For this review, take the finished solid that the model builds, in its own axes (mm). Round coordinates to 2 decimals unless told otherwise and drop trailing zeros. Order: outer loops, then holes, each group sorted by start corner. A loop starts at its lowest first (then second) coordinate and runs counter-clockwise, first axis right, second up. Notation, with made-up numbers: M 2.5,-23 L 6.5,-23 A12 ccw 6.5,-7 Z; hole C 81.25,-35 d2. An arc over 180 degrees is marked long. Write item = value, one per line. Start each with the question number.
from build123d import *

# Parameters (mm, degrees)
SKETCH1_R           = 109
BOSS_EXTRUDE1_DEPTH = 5
SKETCH2_R           = 114
SKETCH2_R_2         = 109
BOSS_EXTRUDE2_DEPTH = 105.1
SKETCH3_R           = 114
BOSS_EXTRUDE3_DEPTH = 5


with BuildPart() as part:
    # Sketch1 → Boss-Extrude1 (new body)
    with BuildSketch(Plane(origin=(0, 0, 0), x_dir=(1, 0, 0), z_dir=(0, 1, 0))):
        with BuildLine():
            Line((-299.6, 119.999333331), (0.396666667, 118.999338887))
            ThreePointArc((0.396666667, 118.999338887), (119, 0), (0.396666667, -118.999338887))
            Line((0.396666667, -118.999338887), (-299.6, -119.999333331))
            ThreePointArc((-299.6, -119.999333331), (-420, 0), (-299.6, 119.999333331))
        make_face()
        with BuildLine():
            ThreePointArc((0.38, -113.999366665), (114, 0), (0.38, 113.999366665))
            Line((0.38, 113.999366665), (-299.616666667, 114.999361109))
            ThreePointArc((-299.616666667, 114.999361109), (-415, 0), (-299.616666667, -114.999361109))
            Line((-299.616666667, -114.999361109), (0.38, -113.999366665))
        make_face(mode=Mode.SUBTRACT)
        with BuildLine():
            Line((0.38, -113.999366665), (-299.616666667, -114.999361109))
            ThreePointArc((-299.616666667, -114.999361109), (-415, 0), (-299.616666667, 114.999361109))
            Line((-299.616666667, 114.999361109), (0.38, 113.999366665))
            ThreePointArc((0.38, 113.999366665), (114, 0), (0.38, -113.999366665))
        make_face()
        with Locations(Location((0, 0, 0), (0, 0, 270))):
            Circle(SKETCH1_R, mode=Mode.SUBTRACT)
    extrude(amount=BOSS_EXTRUDE1_DEPTH)

    # Sketch2 → Boss-Extrude2 (add)
    with BuildSketch(Plane(origin=(0, 5, 0), x_dir=(1, 0, 0), z_dir=(0, 1, 0))):
        with Locations(Location((0, 0, 0), (0, 0, 270))):
            Circle(SKETCH2_R)
        with Locations(Location((0, 0, 0), (0, 0, 270))):
            Circle(SKETCH2_R_2, mode=Mode.SUBTRACT)
    extrude(amount=BOSS_EXTRUDE2_DEPTH)

    # Sketch3 → Boss-Extrude3 (add)
    with BuildSketch(Plane(origin=(0, 110.1, 0), x_dir=(1, 0, 0), z_dir=(0, 1, 0))):
        with Locations(Location((0, 0, 0), (0, 0, 270))):
            Circle(SKETCH3_R)
    extrude(amount=BOSS_EXTRUDE3_DEPTH)


solid = part.part
(1) Draft analysis for pull direction Z (two halves, no side actions). For faces 1 (the cylindrical face through (-111.29, 59.28, -24.71)), 2 (the cylindrical face through (-106.408, 54.279, -23.629)), 3 (the flat face through (-207, 0, -2)), 4 (the flat face through (2, 110.1, -2)), state which applies: released by +Z, released by -Z, zero draft, split by the parting line, or undercut.
(2) We need section B-B, the plane y = 15. Write out the cut boundary in (x, z), then the cut area to 3 significant figures.
(3) We need section C-C, the plane z = -53.5. Write out the cut boundary in (x, y).
(4) Insertion check: pin 1 (1 mm diameter, centred on y = 83, z = -9, fed in from +X); pin 2 (8 mm diameter, centred on y = 81, z = -94.5, fed in from -X); pin 3 (10 mm diameter, centred on x = -256, z = 56, fed in from +Y). Each pin has a flat end and moves straight along its axis. Give the tip position at first contact, or say it passes through.
(5) We need section D-D, the plane x = -120. Write out the cut boundary in (y, z), then the cut area to 3 significant figures.
(6) We need section A-A, the plane z = 0. Write out the cut boundary in (x, y).
(7) For line 1 along X through (y, z) = (76, 0); line 2 along Y through (x, z) = (-137, 4.5); line 3 along Y through (x, z) = (-29, 37.5), list the stretches that pass through material, from the lowest coordinate up.
Values:
q1.face_1 = split by the parting line
q1.face_2 = undercut
q1.face_3 = zero draft
q1.face_4 = undercut
q2.outline = C 0,0 d228; hole C 0,0 d218
q2.area = 3,500 mm²
q3.outline = M -407.41,0 L -94.97,0 L -94.97,110.1 L 94.97,110.1 L 94.97,0 L 106.3,0 L 106.3,5 L 100.67,5 L 100.67,115.1 L -100.67,115.1 L -100.67,5 L -407.41,5 Z
q4.pin_1 = 113.68
q4.pin_2 = -69.32
q4.pin_3 = 5
q5.outline = M 0,-119.4 L 5,-119.4 L 5,119.4 L 0,119.4 Z
q5.area = 1,190 mm²
q6.outline = M -420,0 L -109,0 L -109,110.1 L 109,110.1 L 109,0 L 119,0 L 119,5 L 114,5 L 114,115.1 L -114,115.1 L -114,5 L -420,5 Z
q7.line_1 = -114 to -109, 109 to 114
q7.line_2 = 0 to 5
q7.line_3 = 110.1 to 115.1
